from build123d import *

# Parameters (mm, degrees)
BASE_EXTRUDE_DEPTH  = 5
SKETCH12_R          = 1.5
CUT_EXTRUDE11_DEPTH = 10
BOSS_EXTRUDE1_DEPTH = 25
CUT_EXTRUDE14_DEPTH = 20
CUT_EXTRUDE15_DEPTH = 20
SKETCH15_R          = 2.75
CUT_EXTRUDE16_DEPTH = 20
SKETCH16_R          = 2.5
EXTRUDE1_DEPTH      = 10
SKETCH17_R          = 2.75
EXTRUDE2_DEPTH      = 6


with BuildPart() as part:
    # Sketch1 → Base-Extrude (new body)
    with BuildSketch(Plane.XY):
        Polygon((-27.670446838, -25.657666931), (-27.670446838, -38.157666931), (-20.170446838, -45.657666931), (-12.670446838, -45.657666931), (-12.670446838, -90.657666931), (-32.670446838, -90.657666931), (-37.670446838, -96.707666931), (-42.670446838, -90.657666931), (-62.670446838, -90.657666931), (-62.670446838, -63.157666931), (-68.719237079, -58.157666931), (-62.670446838, -53.157666931), (-62.670446838, -25.657666931), align=None)
    extrude(amount=BASE_EXTRUDE_DEPTH)

    # Sketch12 → Cut-Extrude11 (cut)
    with BuildSketch(Plane.XY.offset(5)):
        with Locations((-65.219237079, -58.157666931)):
            Circle(SKETCH12_R)
        with Locations((-37.670446838, -93.207666931)):
            Circle(SKETCH12_R)
        with Locations((-25.195573104, -43.182793197)):
            Circle(SKETCH12_R)
    extrude(amount=-CUT_EXTRUDE11_DEPTH, mode=Mode.SUBTRACT)

    # Sketch13 → Boss-Extrude1 (add)
    with BuildSketch(Plane.XY.offset(5)):
        Polygon((-62.670446838, -25.657666931), (-62.670446838, -90.657666931), (-12.670446838, -90.657666931), (-12.670446838, -45.657666931), (-27.670446838, -45.657666931), (-27.670446838, -25.657666931), align=None)
    extrude(amount=BOSS_EXTRUDE1_DEPTH)

    # Sketch2 → Cut-Extrude14 (cut)
    with BuildSketch(Plane.XY.offset(5)):
        Polygon((-57.670446838, -55.511686018), (-57.670446838, -60.803647844), (-57.670446838, -85.657666931), (-40.31612782, -85.657666931), (-35.024765855, -85.657666931), (-17.670446838, -85.657666931), (-17.670446838, -50.657666931), (-22.24151465, -50.657666931), (-32.670446838, -50.657666931), (-32.670446838, -40.228734743), (-32.670446838, -30.657666931), (-57.670446838, -30.657666931), align=None)
    extrude(amount=-CUT_EXTRUDE14_DEPTH, mode=Mode.SUBTRACT)

    # Sketch14 → Cut-Extrude15 (cut)
    with BuildSketch(Plane(origin=(0, 0, 5), x_dir=(-1, 0, 0), z_dir=(0, 0, -1))):
        Polygon((32.670446838, -30.657666931), (57.670446838, -30.657666931), (57.670446838, -85.657666931), (17.670446838, -85.657666931), (17.670446838, -50.657666931), (32.670446838, -50.657666931), align=None)
    extrude(amount=-CUT_EXTRUDE15_DEPTH, mode=Mode.SUBTRACT)

    # Sketch15 → Cut-Extrude16 (cut)
    with BuildSketch(Plane.XY.offset(30)):
        with Locations((45, -75.657666931)):
            Circle(SKETCH15_R)
        with Locations((-42, -78)):
            Circle(SKETCH15_R)
    extrude(amount=-CUT_EXTRUDE16_DEPTH, mode=Mode.SUBTRACT)

    # Sketch16 → Extrude1 (cut)
    with BuildSketch(Plane(origin=(-12.670446838, 0, 0), x_dir=(0, 0, -1), z_dir=(1, 0, 0))):
        with Locations((0, -75.65766693)):
            Circle(SKETCH16_R)
    extrude(amount=-EXTRUDE1_DEPTH, mode=Mode.SUBTRACT)

    # Sketch17 → Extrude2 (cut)
    with BuildSketch(Plane(origin=(0, 0, 25), x_dir=(-1, 0, 0), z_dir=(0, 0, -1))):
        with Locations((42, -37)):
            Circle(SKETCH17_R)
    extrude(amount=-EXTRUDE2_DEPTH, mode=Mode.SUBTRACT)


solid = part.part
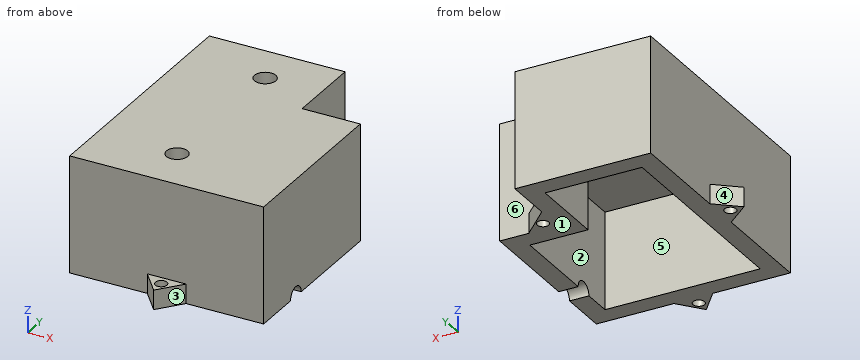
Can you work these out from the model? Positions are in its coordinate system, mm. Face numbers are marked on the shaded views. A direction names the side the tool comes from. Coordinates: 2 decimals unless noted, no trailing zeros. Loops run counter-clockwise (first coordinate to the right, second up) from the corner with the lowest first, then second, coordinate; pieces in that order, holes last. Notation, with made-up numbers: (77, 20) - (131, 20) arc R22 ccw to (131, 46) - close; hole circle Ø7 at (41.5, 23.5). An arc over 180 degrees is marked (long way). Answer as a JSON object with one key per item and string values. Group by question number.
Item 1: If we section it at B-B (x = -18.5): List the corners of the cut face in (y, z) for me, plus the area to 3 significant figures.
Item 2: On a 3-axis mill with a long thin cutter (end or side, diameter ignored), from which of +Z, -Z, +X, -X, +Y, -Y can I reach the whole of each face in a straight line? I mean the marked faces 4, 5 and 6. Say none if no direction works.
Item 3: For pin 1 (4 mm diameter, centred on x = -37.67, y = -93.21, fed in from +Z); pin 2 (2 mm diameter, centred on x = -30.5, z = 14.5, fed in from -Y); pin 3 (10 mm diameter, centred on x = -29, y = -59.5, fed in from -Z), each with a flat end and sliding along its axis, tell me the tip position at first contact or that it passes through.
Item 4: If we section it at A-A (y = -37): List the corners of the cut face in (x, z) for me.
Item 5: If I drill on L1, parallel to Y at x = -39.5, z = 20.5; L2, parallel to X at y = -32, z = 5; L3, parallel to Y at x = -42, z = 26.95, over which ranges is the centre line in solid material (lowest first)? Write a range as from..to.
Item 6: If we section it at C-C (z = 14.5): List the corners of the cut face in (x, y) for me.
Item 7: If we section it at D-D (y = -70.5): List the corners of the cut face in (x, z) for me, plus the area to 3 significant figures.
Item 8: If we mould it in two halves opening along Y, with no side actions, what happens to the marked faces 1, 2 and 3? For each: released by +Y, released by -Y, zero draft, split by the parting line, or undercut.
Returned:
{
 "1": {"outline": "(-90.66, 0) - (-85.66, 0) - (-85.66, 25) - (-50.66, 25) - (-50.66, 0) - (-45.66, 0) - (-45.66, 30) - (-90.66, 30) - close", "area": "475 mm²"},
 "2": {"face 4": "+Z, -Z, -X, +Y", "face 5": "-Z", "face 6": "+Z, +X, +Y"},
 "3": {"pin 1": "stops at z = 5", "pin 2": "stops at y = -90.66", "pin 3": "stops at z = 25"},
 "4": {"outline": "(-62.67, 0) - (-57.67, 0) - (-57.67, 25) - (-44.75, 25) - (-44.75, 30) - (-62.67, 30) - close; (-39.25, 25) - (-32.67, 25) - (-32.67, 0) - (-27.67, 0) - (-27.67, 30) - (-39.25, 30) - close"},
 "5": {"L1": "y = -90.66..-85.66, -30.66..-25.66", "L2": "x = -62.67..-57.67, -32.67..-27.67", "L3": "y = -90.66..-80.75, -75.25..-39.75, -34.25..-25.66"},
 "6": {"outline": "(-62.67, -90.66) - (-12.67, -90.66) - (-12.67, -45.66) - (-27.67, -45.66) - (-27.67, -25.66) - (-62.67, -25.66) - close; hole (-57.67, -85.66) - (-17.67, -85.66) - (-17.67, -50.66) - (-32.67, -50.66) - (-32.67, -30.66) - (-57.67, -30.66) - close"},
 "7": {"outline": "(-62.67, 0) - (-57.67, 0) - (-57.67, 25) - (-17.67, 25) - (-17.67, 0) - (-12.67, 0) - (-12.67, 30) - (-62.67, 30) - close", "area": "500 mm²"},
 "8": {"face 1": "zero draft", "face 2": "undercut", "face 3": "released by -Y"}
}
